```python
from build123d import *

# Parameters (mm, degrees)
F0_W     = 25
F0_H     = 25
F1_DEPTH = 25
F3_D     = 6
F5_D     = 5
F7_D     = 5


with BuildPart() as f1:
    # F0 (on Top) → F1 (new body)
    with BuildSketch(Plane.XY):
        with Locations((-12.5, 12.5)):
            Rectangle(F0_W, F0_H)
    extrude(amount=F1_DEPTH)

    # F3 (through all)
    with Locations(Plane.XY.offset(25)):
        with Locations((-12.5, 12.5)):
            Hole(F3_D / 2)

    # F5 (through all)
    with Locations(Plane.XZ):
        with Locations((-12.5, 20)):
            Hole(F5_D / 2)

    # F7 (through all)
    with Locations(Plane.XZ):
        with Locations((-12.5, 5)):
            Hole(F7_D / 2)


solid = f1.part
```
Geometry: final body of the model. Coordinates: model frame, mm. Coordinates: 2 decimals unless noted, no trailing zeros. Order: outer loops, then holes, each group sorted by start corner. A loop starts at its lowest first (then second) coordinate and runs counter-clockwise, first axis right, second up.
Item 1: Draft query along Y for faces 1 (the face through (-13.884, 9.838, 12.325)), 2 (the face through (-13, 25, 12)), 3 (the face through (0, 12, 12)). Return one class per face: released by +Y, released by -Y, zero draft, split by the parting line, or undercut.
Answer:
face 1: undercut
face 2: released by +Y
face 3: zero draft
Item 2: Section query A-A (y = 12.5). Output: boundary loops of the cut face in (x, z).
Answer:
outline: (-25, 0) - (-15.5, 0) - (-15.5, 25) - (-25, 25) - close; (-9.5, 0) - (0, 0) - (0, 25) - (-9.5, 25) - close
Item 3: Section query C-C (z = 20). Output: boundary loops of the cut face in (x, y), then the cut area to 3 significant figures.
Answer:
outline: (-25, 0) - (-15, 0) - (-15, 10.84) arc R3 cw to (-15, 14.16) - (-15, 25) - (-25, 25) - close; (-10, 0) - (0, 0) - (0, 25) - (-10, 25) - (-10, 14.16) arc R3 cw to (-10, 10.84) - close
area: 498 mm2
Item 4: Material intervals for line 1 along Z through (x, y) = (-12.5, 7.5); line 2 along X through (y, z) = (16.75, 5); line 3 along Z through (x, y) = (-11.75, 22.5), sorted ascending.
Answer:
line 1: z = 0 to 2.5, 7.5 to 17.5, 22.5 to 25
line 2: x = -25 to -15, -10 to 0
line 3: z = 0 to 2.62, 7.38 to 17.62, 22.38 to 25
Item 5: Section query B-B (x = -12.5). Output: boundary loops of the cut face in (y, z), then the cut area to 3 significant figures.
Answer:
outline: (0, 0) - (9.5, 0) - (9.5, 2.5) - (0, 2.5) - close; (0, 7.5) - (9.5, 7.5) - (9.5, 17.5) - (0, 17.5) - close; (0, 22.5) - (9.5, 22.5) - (9.5, 25) - (0, 25) - close; (15.5, 0) - (25, 0) - (25, 2.5) - (15.5, 2.5) - close; (15.5, 7.5) - (25, 7.5) - (25, 17.5) - (15.5, 17.5) - close; (15.5, 22.5) - (25, 22.5) - (25, 25) - (15.5, 25) - close
area: 285 mm2
Item 6: Section query D-D (z = 16.5). Output: boundary loops of the cut face in (x, y).
Answer:
outline: (-25, 0) - (0, 0) - (0, 25) - (-25, 25) - close; hole circle Ø6 at (-12.5, 12.5)
